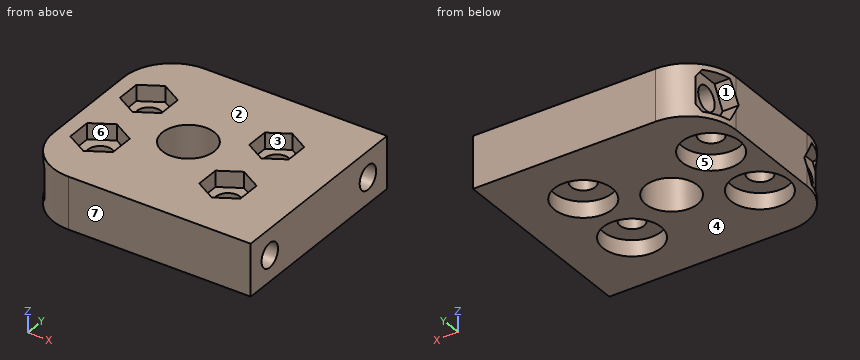
from build123d import *

# Parameters (mm, degrees)
SKETCH008_W     = 57.65
SKETCH008_H     = 50
PAD_DEPTH       = 13
SKETCH009_R     = 3.015
POCKET_DEPTH    = 23.501
FILLET_R        = 12
SKETCH_R        = 6.5
POCKET001_DEPTH = 13.001
POCKET002_DEPTH = 4
SKETCH011_R     = 7.25
POCKET003_DEPTH = 4
SKETCH012_R     = 3.015
POCKET004_DEPTH = 57.651
POCKET005_DEPTH = 4


with BuildPart() as part:
    # Sketch008 → Pad (new body)
    with BuildSketch(Plane.XY):
        with Locations((3.825, 0)):
            Rectangle(SKETCH008_W, SKETCH008_H)
    extrude(amount=PAD_DEPTH)

    # Sketch009 → Pocket (cut, through all)
    with BuildSketch(Plane.XY.offset(23.5)):
        with Locations((-16, 8.955)):
            Circle(SKETCH009_R)
        with Locations((-16, -8.955)):
            Circle(SKETCH009_R)
        with Locations((16, 8.955)):
            Circle(SKETCH009_R)
        with Locations((16, -8.955)):
            Circle(SKETCH009_R)
    extrude(amount=-POCKET_DEPTH, mode=Mode.SUBTRACT)

    # Fillet
    fillet_edges = [part.edges().sort_by_distance(p)[0] for p in [
        (-25, 25, 6.5),
        (-25, -25, 6.5),
    ]]
    fillet(fillet_edges, radius=FILLET_R)

    # Sketch (on Face5 of Fillet) → Pocket001 (cut, through all)
    with BuildSketch(Plane.XY.offset(13)):
        Circle(SKETCH_R)
    extrude(amount=-POCKET001_DEPTH, mode=Mode.SUBTRACT)

    # Sketch010 (on Face5 of Pocket001) → Pocket002 (cut)
    with BuildSketch(Plane.XY.offset(13)):
        Polygon((-10.8, 11.957221), (-16, 14.959443), (-21.2, 11.957221), (-21.2, 5.952779), (-16, 2.950557), (-10.8, 5.952779), align=None)
        Polygon((20.944817, 11.809891), (16, 14.664783), (11.055183, 11.809891), (11.055183, 6.100109), (16, 3.245217), (20.944817, 6.100109), align=None)
        Polygon((-10.662676, -5.873494), (-16, -2.791989), (-21.337324, -5.873494), (-21.337324, -12.036506), (-16, -15.118011), (-10.662676, -12.036506), align=None)
        Polygon((21.146526, -5.983652), (16, -3.012303), (10.853474, -5.983652), (10.853474, -11.926348), (16, -14.897697), (21.146526, -11.926348), align=None)
    extrude(amount=-POCKET002_DEPTH, mode=Mode.SUBTRACT)

    # Sketch011 (on Face2 of Pocket002) → Pocket003 (cut)
    with BuildSketch(Plane(origin=(0, 0, 0), x_dir=(1, 0, 0), z_dir=(0, 0, -1))):
        with Locations((-16, 8.955)):
            Circle(SKETCH011_R)
        with Locations((16, 8.955)):
            Circle(SKETCH011_R)
        with Locations((-16, -8.955)):
            Circle(SKETCH011_R)
        with Locations((16, -8.955)):
            Circle(SKETCH011_R)
    extrude(amount=-POCKET003_DEPTH, mode=Mode.SUBTRACT)

    # Sketch012 (on Face4 of Pocket003) → Pocket004 (cut, through all)
    with BuildSketch(Plane.YZ.offset(32.65)):
        with Locations((18, 6.5)):
            Circle(SKETCH012_R)
        with Locations((-18, 6.5)):
            Circle(SKETCH012_R)
    extrude(amount=-POCKET004_DEPTH, mode=Mode.SUBTRACT)

    # Sketch013 (on Face6 of Pocket004) → Pocket005 (cut)
    with BuildSketch(Plane(origin=(-25, 0, 0), x_dir=(0, -1, 0), z_dir=(-1, 0, 0))):
        Polygon((-12.053292, 6.5), (-15.026646, 11.65), (-20.973354, 11.65), (-23.946708, 6.5), (-20.973354, 1.35), (-15.026646, 1.35), align=None)
        Polygon((23.946708, 6.5), (20.973354, 11.65), (15.026646, 11.65), (12.053292, 6.5), (15.026646, 1.35), (20.973354, 1.35), align=None)
    extrude(amount=-POCKET005_DEPTH, mode=Mode.SUBTRACT)


solid = part.part
For this review, take the finished solid that the model builds, in its own axes (mm). Face numbers are marked on the shaded views. A direction names the side the tool comes from. Round coordinates to 2 decimals unless told otherwise and drop trailing zeros. Write each loop counter-clockwise with the first axis right and the second up, starting at its lowest first coordinate (ties: lowest second). Pieces come first, ordered by that corner, then holes. Notation, with made-up numbers: (37.5, -14) - (42.5, -14) arc R26 ccw to (42.5, 10) - close; hole circle Ø1 at (71.25, 20). An arc over 180 degrees is marked (long way). Use a Markdown table: item, result.
Q1. We need section C-C (z = 7.25). Give the boundary of the cut face in (x, y) (3 decimals), plus the area to 3 significant figures.
Derived:
| item | result |
|---|---|
| outline | (-25, -12.486) - (-21, -12.486) - (-21, -15.08) - (32.65, -15.08) - (32.65, 15.08) - (-21, 15.08) - (-21, 12.486) - (-25, 12.486) - close; (-21, -21.944) arc R12 ccw to (-13, -25) - (32.65, -25) - (32.65, -20.92) - (-21, -20.92) - close; (-21, 20.92) - (32.65, 20.92) - (32.65, 25) - (-13, 25) arc R12 ccw to (-21, 21.944) - close; hole circle Ø6.03 at (-16, -8.955); hole circle Ø6.03 at (-16, 8.955); hole circle Ø13 at (0, 0); hole circle Ø6.03 at (16, -8.955); hole circle Ø6.03 at (16, 8.955) |
| area | 1,890 mm2 |
Q2. The part is to be moulded in two halves that separate along Z. For the marked faces 1, 2, 3 and 4, say which applies: pulls with the +Z half, pulls with the -Z half, needs draft (parallel to the pull), parting line crosses it, or undercut.
Derived:
| item | result |
|---|---|
| face 1 | undercut |
| face 2 | pulls with the +Z half |
| face 3 | needs draft |
| face 4 | pulls with the -Z half |
Q3. Machinability: for the marked faces 5, 6 and 7, which of the approach directions +Z, -Z, +X, -X, +Y, -Y give a long, thin tool a straight path to every point of the face, cutting with its end or side? Answer none if there is none.
Derived:
| item | result |
|---|---|
| face 5 | -Z |
| face 6 | +Z |
| face 7 | +Z, -Z, +X, -X, -Y |
Q4. Wall thickness on line 1 along Y through (x, z) = (16, 1.1) (3 decimals); line 2 along X through (y, z) = (8, 10); line 3 along X through (y, z) = (-8, 11): over which ranges is each line inside the solid? List them lowest first.
Derived:
| item | result |
|---|---|
| line 1 | y = -25 to -16.205, -1.705 to 1.705, 16.205 to 25 |
| line 2 | x = -25 to -21.2, -10.8 to 11.06, 20.94 to 32.65 |
| line 3 | x = -25 to -21.34, -10.66 to 10.85, 21.15 to 32.65 |
Q5. We need section B-B (y = 0). Give the boundary of the cut face in (x, z), plus the area to 3 significant figures.
Derived:
| item | result |
|---|---|
| outline | (-25, 0) - (-6.5, 0) - (-6.5, 13) - (-25, 13) - close; (6.5, 0) - (32.65, 0) - (32.65, 13) - (6.5, 13) - close |
| area | 580 mm2 |
Q6. We need section D-D (y = -8). Give the boundary of the cut face in (x, z).
Derived:
| item | result |
|---|---|
| outline | (-25, 0) - (-23.19, 0) - (-23.19, 4) - (-18.86, 4) - (-18.86, 9) - (-21.34, 9) - (-21.34, 13) - (-25, 13) - close; (-13.14, 4) - (-8.81, 4) - (-8.81, 0) - (8.81, 0) - (8.81, 4) - (13.14, 4) - (13.14, 9) - (10.85, 9) - (10.85, 13) - (-10.66, 13) - (-10.66, 9) - (-13.14, 9) - close; (18.86, 4) - (23.19, 4) - (23.19, 0) - (32.65, 0) - (32.65, 13) - (21.15, 13) - (21.15, 9) - (18.86, 9) - close |
Q7. We need section A-A (x = 0). Give the boundary of the cut face in (y, z) (3 decimals), plus the area to 3 significant figures.
Derived:
| item | result |
|---|---|
| outline | (-25, 0) - (-6.5, 0) - (-6.5, 13) - (-25, 13) - close; (6.5, 0) - (25, 0) - (25, 13) - (6.5, 13) - close; hole circle Ø6.03 at (-18, 6.5); hole circle Ø6.03 at (18, 6.5) |
| area | 424 mm2 |
Q8. Clearance check with flat-ended pins moving along their axes: pin 1 (11.5 mm diameter, centred on x = -16, y = 8.5, fed in from -Z); pin 2 (5 mm diameter, centred on x = -16, y = 10, fed in from +Z). State where each tip first meets the part, or that it passes through.
Derived:
| item | result |
|---|---|
| pin 1 | stops at z = 4 |
| pin 2 | stops at z = 9 |
